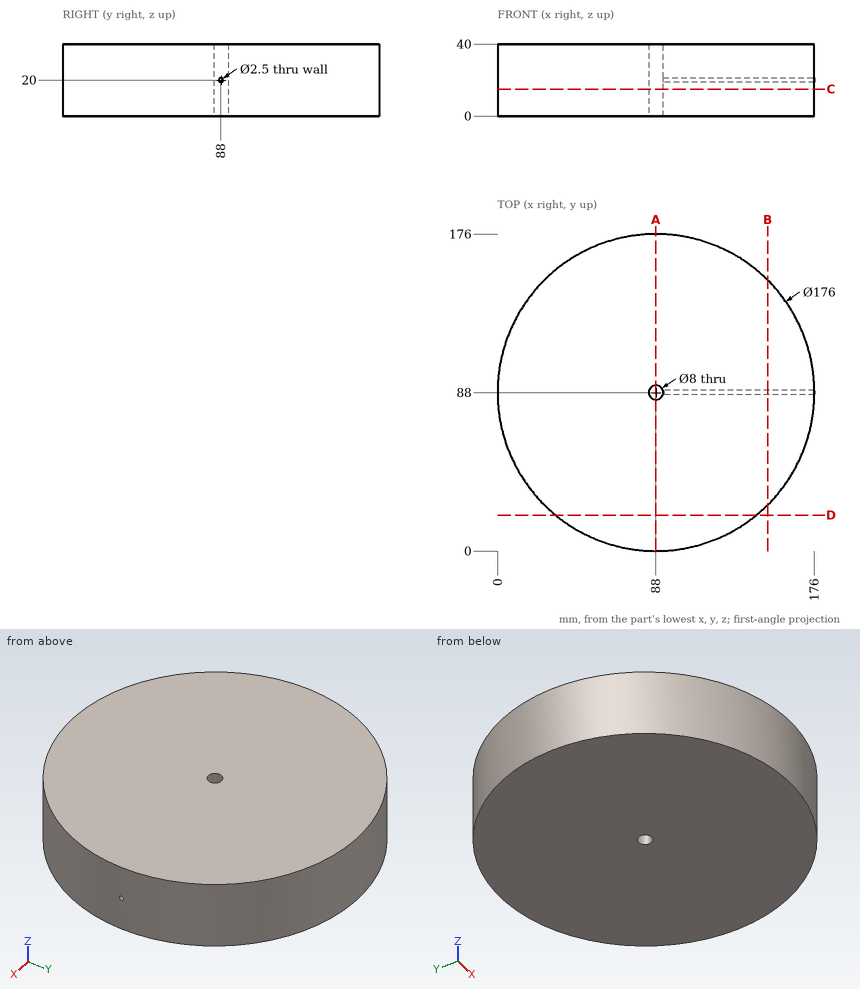
Geometry: see drawing. Coordinates: mm, zero at the bounding-box minimum. Round coordinates to 2 decimals unless told otherwise and drop trailing zeros. Loops run counter-clockwise (first coordinate to the right, second up) from the corner with the lowest first, then second, coordinate; pieces in that order, holes last. Notation, with made-up numbers: M -9,77.25 L 19,77.25 A6 cw 19,84.25 Z; hole C 27,41 d4. An arc over 180 degrees is marked long. Use a Markdown table: item, result. Add a question column.
1. Cut plane D-D, the plane y = 20. Output: boundary loops of the cut face in (x, z).
2. Contact query for flat-ended pins moving along their axis: pin 1 (1.5 mm diameter, centred on y = 95, z = 16.5, fed in from +X); pin 2 (2 mm diameter, centred on y = 65, z = 13.5, fed in from +X); pin 3 (1.5 mm diameter, centred on x = 153.5, z = 8, fed in from -Y). Output: stop coordinate, or through.
3. Cut plane C-C, the plane z = 15. Output: boundary loops of the cut face in (x, y), and give its area (3 significant figures).
4. Cut plane B-B, the plane x = 150. Output: boundary loops of the cut face in (y, z).
5. Cut plane A-A, the plane x = 88. Output: boundary loops of the cut face in (y, z).
6. Ray query, line 1 along Y through (x, z) = (88, 26); line 2 along X through (y, z) = (62.5, 30); line 3 along X through (y, z) = (45.5, 11). Return the intervals inside material, ascending. Write a range as [from, to].
Solution:
| question | item | result |
|---|---|---|
| 1 | outline | M 32.14,0 L 143.86,0 L 143.86,40 L 32.14,40 Z |
| 2 | pin 1 | stops at x = 175.78 |
| 2 | pin 2 | stops at x = 173.21 |
| 2 | pin 3 | stops at y = 28.41 |
| 3 | outline | C 88,88 d176; hole C 88,88 d8 |
| 3 | area | 24,300 mm2 |
| 4 | outline | M 25.55,0 L 150.45,0 L 150.45,40 L 25.55,40 Z; hole C 88,20 d2.5 |
| 5 | outline | M 0,0 L 84,0 L 84,40 L 0,40 Z; M 92,0 L 176,0 L 176,40 L 92,40 Z |
| 6 | line 1 | y = [0, 84], [92, 176] |
| 6 | line 2 | x = [3.78, 172.22] |
| 6 | line 3 | x = [10.94, 165.06] |
